Part model, mm, in its own coordinate system. A direction names the side the tool comes from. Round coordinates to 2 decimals unless told otherwise and drop trailing zeros. Loops run counter-clockwise (first coordinate to the right, second up) from the corner with the lowest first, then second, coordinate; pieces in that order, holes last. Notation, with made-up numbers: (26, -32) - (51, -32) arc R25 cw to (51, -2) - close; hole circle Ø5 at (-24, -30.75). An arc over 180 degrees is marked (long way). Write each question's results on one line, items separated by ' | '. Start each with the question number.
(1) Cut at D-D, the plane z = 3.5. List the corners of the cut face in (x, y), then the cut area to 3 significant figures.
(2) Cut at A-A, the plane y = 43. List the corners of the cut face in (x, z).
(3) Cut at B-B, the plane x = 0. List the corners of the cut face in (y, z), then the cut area to 3 significant figures.
(4) Drill centre lines: L1, parallel to Z at x = -15.5, y = 41.5; L2, parallel to X at y = 45, z = -15. Where is each one in solid material? Low to high.
(5) Cut at C-C, the plane y = 26. List the corners of the cut face in (x, z), then the cut area to 3 significant figures.
(6) Tool access for faces 4 (the face through (-21.15, 24, 0)), 5 (the face through (0, 24, 21.15)), 6 (the face through (-18.36, 23.87, -18.29)), 7 (the face through (21.15, 24, 0)), 8 (the face through (-16, 38, 15)): list every direction of +Z, -Z, +X, -X, +Y, -Y with a clear straight run to the whole face (end or side of a thin tool).
(7) Mould opens along Z. For faces 1 (the face through (-17, 43.07, 15.43)), 2 (the face through (18.29, 23.87, -18.36)), 3 (the face through (-18, 15, -19)) say: released by +Z, released by -Z, zero draft, split by the parting line, or undercut.
(8) Flat gauge pins, fed straight in: P1, Ø1.8, axis at x = 15.5, z = 15.5, coming from the +Y side; P2, Ø20, axis at y = 20.5, z = -5, coming from the +X side; P3, Ø6, axis at x = -7, z = 14, coming from the +Y side; P4, Ø2, axis at x = 5.5, z = 10.5, coming from the +Y side. Where does each tip first touch, or does it go through?
from build123d import *

# Parameters (mm, degrees)
BOSS_EXTRUDE1_DEPTH = 48
SKETCH2_R           = 11
BOSS_EXTRUDE2_DEPTH = 2
SKETCH3_R           = 2.5
BOSS_EXTRUDE3_DEPTH = 22
CHAMFER1_SIZE       = 0.5
SKETCH4_R           = 1.5
CUT_EXTRUDE1_DEPTH  = 10
BOSS_EXTRUDE5_DEPTH = 15


with BuildPart() as part:
    # Sketch1 → Boss-Extrude1 (new body)
    with BuildSketch(Plane(origin=(0, 0, 0), x_dir=(1, 0, 0), z_dir=(0, 1, 0))):
        Polygon((15.5, 21.15), (21.15, 15.5), (21.15, -15.5), (15.5, -21.15), (-15.5, -21.15), (-21.15, -15.5), (-21.15, 15.5), (-15.5, 21.15), align=None)
    extrude(amount=BOSS_EXTRUDE1_DEPTH)

    # Sketch2 → Boss-Extrude2 (add)
    with BuildSketch(Plane(origin=(0, 48, 0), x_dir=(1, 0, 0), z_dir=(0, 1, 0))):
        Circle(SKETCH2_R)
    extrude(amount=BOSS_EXTRUDE2_DEPTH)

    # Sketch3 → Boss-Extrude3 (add)
    with BuildSketch(Plane(origin=(0, 50, 0), x_dir=(1, 0, 0), z_dir=(0, 1, 0))):
        Circle(SKETCH3_R)
    extrude(amount=BOSS_EXTRUDE3_DEPTH)

    # Chamfer1
    chamfer1_edges = [part.edges().sort_by_distance(p)[0] for p in [
        (-2.5, 72, 0),
    ]]
    chamfer(chamfer1_edges, length=CHAMFER1_SIZE)

    # Sketch4 → Cut-Extrude1 (cut)
    with BuildSketch(Plane(origin=(0, 48, 0), x_dir=(1, 0, 0), z_dir=(0, 1, 0))):
        with Locations((-15.5, 15.5)):
            Circle(SKETCH4_R)
        with Locations((15.5, 15.5)):
            Circle(SKETCH4_R)
        with Locations((15.5, -15.5)):
            Circle(SKETCH4_R)
        with Locations((-15.5, -15.5)):
            Circle(SKETCH4_R)
    extrude(amount=-CUT_EXTRUDE1_DEPTH, mode=Mode.SUBTRACT)

    # Sketch6 → Boss-Extrude5 (add)
    with BuildSketch(Plane(origin=(0, 48, 0), x_dir=(1, 0, 0), z_dir=(0, 1, 0))):
        Polygon((-21.65, -15.707106781), (-15.707106781, -21.65), (15.707106781, -21.65), (21.65, -15.707106781), (21.65, 15.707106781), (15.707106781, 21.65), (-15.707106781, 21.65), (-21.65, 15.707106781), align=None)
        Polygon((-21.15, -15.5), (-15.5, -21.15), (15.5, -21.15), (21.15, -15.5), (21.15, 15.5), (15.5, 21.15), (-15.5, 21.15), (-21.15, 15.5), align=None, mode=Mode.SUBTRACT)
    boss_extrude5 = extrude(amount=-BOSS_EXTRUDE5_DEPTH)

    # Mirror1: Boss-Extrude5 across plane
    add(boss_extrude5.mirror(Plane.ZX.offset(24)))


solid = part.part
A:
1) outline: (-21.65, 0) - (21.65, 0) - (21.65, 15) - (21.15, 15) - (21.15, 33) - (21.65, 33) - (21.65, 48) - (10.43, 48) - (10.43, 50) - (-10.43, 50) - (-10.43, 48) - (-21.65, 48) - (-21.65, 33) - (-21.15, 33) - (-21.15, 15) - (-21.65, 15) - close | area: 2,100 mm2
2) outline: (-21.65, -15.71) - (-15.71, -21.65) - (15.71, -21.65) - (21.65, -15.71) - (21.65, 15.71) - (15.71, 21.65) - (-15.71, 21.65) - (-21.65, 15.71) - close; hole circle Ø3 at (-15.5, -15.5); hole circle Ø3 at (-15.5, 15.5); hole circle Ø3 at (15.5, -15.5); hole circle Ø3 at (15.5, 15.5)
3) outline: (0, -21.65) - (15, -21.65) - (15, -21.15) - (33, -21.15) - (33, -21.65) - (48, -21.65) - (48, -11) - (50, -11) - (50, -2.5) - (71.5, -2.5) - (72, -2) - (72, 2) - (71.5, 2.5) - (50, 2.5) - (50, 11) - (48, 11) - (48, 21.65) - (33, 21.65) - (33, 21.15) - (15, 21.15) - (15, 21.65) - (0, 21.65) - close | area: 2,210 mm2
4) L1: -21.65 to -17, -14 to 14, 17 to 21.65 | L2: -21.65 to -16.91, -14.09 to 14.09, 16.91 to 21.65
5) outline: (-21.15, -15.5) - (-15.5, -21.15) - (15.5, -21.15) - (21.15, -15.5) - (21.15, 15.5) - (15.5, 21.15) - (-15.5, 21.15) - (-21.15, 15.5) - close | area: 1,730 mm2
6) face 4: +Z, -Z, -X | face 5: +Z, +X, -X | face 6: -Z, -X | face 7: +Z, -Z, +X | face 8: +Y
7) face 1: undercut | face 2: released by -Z | face 3: zero draft
8) P1: y = 38 | P2: x = 21.65 | P3: y = 48 | P4: y = 50
